```python
from build123d import *

# Parameters (mm, degrees)
F1_DEPTH = 101.6
F3_DEPTH = 76.2
F4_W     = 50.8
F4_H     = 25.4
F5_DEPTH = 203.201
F6_W     = 38.1
F6_H     = 38.1
F7_DEPTH = 50.801
F8_R     = 12.7


with BuildPart() as f1:
    # F0 (on Front) → F1 (new body)
    with BuildSketch(Plane.XZ):
        with BuildLine():
            Line((203.2, 0), (0, 0))
            Line((0, 0), (0, -25.4))
            Line((0, -25.4), (38.1, -25.4))
            Line((38.1, -25.4), (38.1, -50.8))
            Line((38.1, -50.8), (63.5, -50.8))
            Line((63.5, -50.8), (63.5, -38.1))
            ThreePointArc((63.5, -38.1), (67.219744, -29.119744), (76.2, -25.4))
            Line((76.2, -25.4), (127, -25.4))
            ThreePointArc((127, -25.4), (135.980256, -29.119744), (139.7, -38.1))
            Line((139.7, -38.1), (139.7, -50.8))
            Line((139.7, -50.8), (165.1, -50.8))
            Line((165.1, -50.8), (165.1, -25.4))
            Line((165.1, -25.4), (203.2, -25.4))
            Line((203.2, -25.4), (203.2, 0))
        make_face()
    extrude(amount=F1_DEPTH)

    # F2 (on Top) → F3 (join)
    with BuildSketch(Plane.XY):
        Polygon((152.4, 0), (50.8, 0), (101.6, -101.6), align=None)
    extrude(amount=F3_DEPTH)

    # F4 (on Right) → F5 (cut, through all)
    with BuildSketch(Plane.YZ):
        with Locations((-76.2, 38.1)):
            Rectangle(F4_W, F4_H)
    extrude(amount=F5_DEPTH, mode=Mode.SUBTRACT)

    # F6 (on Top) → F7 (cut, through all)
    with BuildSketch(Plane.XY):
        with Locations((19.05, -50.8)):
            Rectangle(F6_W, F6_H)
        with Locations((184.15, -50.8)):
            Rectangle(F6_W, F6_H)
    extrude(amount=-F7_DEPTH, mode=Mode.SUBTRACT)

    # F8
    f8_edges = [f1.edges().sort_by_distance(p)[0] for p in [
        (0, -101.6, -12.7),
        (0, 0, -12.7),
        (203.2, 0, -12.7),
        (203.2, -101.6, -12.7),
    ]]
    fillet(f8_edges, radius=F8_R)


solid = f1.part
```
Design review of the part built by this model. Coordinates are the model's own, in mm. A direction names the side the tool comes from. Give positions to 0.01 mm unless a question says otherwise; leave off trailing zeros. Order: outer loops, then holes, each group sorted by start corner. A loop starts at its lowest first (then second) coordinate and runs counter-clockwise, first axis right, second up. Notation, with made-up numbers: (-0.5, 2.25) -> (24.5, 2.25) arc R5 ccw to (24.5, 7.25) -> close; hole circle Ø4 at (43.25, 65). An arc over 180 degrees is marked (long way). Write each question's results on one line, items separated by ' | '. Start each with the question number.
Q1. Mouldability with a two-part tool opening along Y and no side actions: class faces 1 (the flat face through (100, 0, 14)), 2 (the flat face through (101, -71, 50.8)), 3 (the cylindrical face through (199.58, -97.78, -12.52)), 4 (the flat face through (19, -31.75, -13)) as +Y half, -Y half, draft (parallel to the pull), parting line (faces both ways), or undercut.
Q2. Add section D-D on x = 93. Give the boundary of the cut face in (y, z), and give its area (3 significant figures).
Q3. Add section A-A on x = 22. Give the boundary of the cut face in (y, z), and give its area (3 significant figures).
Q4. Machinability: for faces 5 (the cylindrical face through (67.12, -50.09, -29.22)), 6 (the flat face through (164, -61, 0)), 7 (the flat face through (19, -86, -25.4)), 8 (the flat face through (184, -69.85, -13)), which of the approach directions +Z, -Z, +X, -X, +Y, -Y give a long, thin tool a straight path to every point of the face, cutting with its end or side? Answer none if there is none.
Q5. For pin 1 (3 mm diameter, centred on x = 122.5, z = 20.5, fed in from -Y); pin 2 (7.5 mm diameter, centred on x = 110, z = 39, fed in from -Y); pin 3 (8 mm diameter, centred on y = -40, z = -7.5, fed in from -X), all flat-tipped, find the tip position at first contact; note any pin that passes through.
Q6. Wall thickness on L1, parallel to X at y = -74, z = -45.5; L2, parallel to Y at x = 20, z = -12.5; L3, parallel to Z at x = 47, y = -34.5: over which ranges is each line inside the solid? List them lowest first. Write a range as from..to.
Q7. Add section B-B on y = -65.5. Give the boundary of the cut face in (x, z).
Q8. Add section C-C on z = -31. Give the boundary of the cut face in (x, y), and give its area (3 significant figures).
Found:
1) face 1: +Y half | face 2: draft | face 3: -Y half | face 4: undercut
2) outline: (-101.6, -25.4) -> (0, -25.4) -> (0, 76.2) -> (-84.4, 76.2) -> (-84.4, 50.8) -> (-50.8, 50.8) -> (-50.8, 25.4) -> (-84.4, 25.4) -> (-84.4, 0) -> (-101.6, 0) -> close | area: 8,160 mm2
3) outline: (-101.6, -25.4) -> (-69.85, -25.4) -> (-69.85, 0) -> (-101.6, 0) -> close; (-31.75, -25.4) -> (0, -25.4) -> (0, 0) -> (-31.75, 0) -> close | area: 1,610 mm2
4) face 5: -Z, +Y, -Y | face 6: +Z, +X, -Y | face 7: -Z, -X, +Y, -Y | face 8: +Z, -Z, +X
5) pin 1: stops at y = -62.8 | pin 2: stops at y = -50.8 | pin 3: stops at x = 38.1
6) L1: x = 38.1..63.5, 139.7..165.1 | L2: y = -101.6..-69.85, -31.75..0 | L3: z = -50.8..0
7) outline: (38.1, -50.8) -> (63.5, -50.8) -> (63.5, -38.1) arc R12.7 cw to (76.2, -25.4) -> (127, -25.4) arc R12.7 cw to (139.7, -38.1) -> (139.7, -50.8) -> (165.1, -50.8) -> (165.1, 0) -> (119.65, 0) -> (119.65, 25.4) -> (83.55, 25.4) -> (83.55, 0) -> (38.1, 0) -> close; (83.55, 50.8) -> (119.65, 50.8) -> (119.65, 76.2) -> (83.55, 76.2) -> close
8) outline: (38.1, -101.6) -> (65.67, -101.6) -> (65.67, 0) -> (38.1, 0) -> close; (137.53, -101.6) -> (165.1, -101.6) -> (165.1, 0) -> (137.53, 0) -> close | area: 5,600 mm2
